Can you work these out from the model? Positions are in its coordinate system, mm. A direction names the side the tool comes from. Round coordinates to 2 decimals unless told otherwise and drop trailing zeros. Loops run counter-clockwise (first coordinate to the right, second up) from the corner with the lowest first, then second, coordinate; pieces in that order, holes last.
(1) Which directions (+Z, -Z, +X, -X, +Y, -Y) give clear straight access to the entire face, cutting with the end or side of a thin tool? Please do faces 1 (the face through (116, 29, 60)), 2 (the face through (62.57, 42.85, 1.18)), 3 (the face through (112, 26, 33.6)).
(2) I want a section at C-C on x = 49. Write out the boundary of the cut face in (y, z), plus the area to 3 significant figures.
(3) Will these pins go through, and if not, where does the flat tip stop? pin 1 Ø4 at (x, z) = (110.5, 112.5) entering from +Y; pin 2 Ø1.5 at (x, z) = (69.5, 46.5) entering from +Y.
(4) If I drill on line 1 along Z through (x, y) = (45.5, 32.5); line 2 along Y through (x, z) = (52, 1.25); line 3 along X through (y, z) = (12, 83), over which ranges is the centre line in solid material (lowest first)?
(5) Thinking about a two-plate mould opening in Z: for faces 4 (the face through (2, 58.4, 32)), 5 (the face through (7.2, 26, 114)), which applies, released by +Z, released by -Z, zero draft, split by the parting line, or undercut?
(6) I want a section at B-B on z = 105.5. Write out the boundary of the cut face in (x, y), plus the area to 3 significant figures.
from build123d import *

# Parameters (mm, degrees)
SKETCH1_W           = 116
SKETCH1_H           = 117.6
BOSS_EXTRUDE1_DEPTH = 2.4
SKETCH2_W           = 116
SKETCH2_H           = 117.6
SKETCH2_W_2         = 111.2
SKETCH2_H_2         = 112.8
BOSS_EXTRUDE2_DEPTH = 56
SKETCH3_R           = 1.5
CUT_EXTRUDE1_DEPTH  = 10
SKETCH7_W           = 4.8
SKETCH7_H           = 4.8
BOSS_EXTRUDE4_DEPTH = 45.6
FILLET2_R           = 2
SKETCH8_R           = 6
CUT_EXTRUDE2_DEPTH  = 10


with BuildPart() as part:
    # Sketch1 → Boss-Extrude1 (new body)
    with BuildSketch(Plane(origin=(0, 0, 0), x_dir=(1, 0, 0), z_dir=(0, 1, 0))):
        with Locations((58, -58.8)):
            Rectangle(SKETCH1_W, SKETCH1_H)
    extrude(amount=BOSS_EXTRUDE1_DEPTH)

    # Sketch2 → Boss-Extrude2 (add)
    with BuildSketch(Plane(origin=(0, 2.4, 0), x_dir=(1, 0, 0), z_dir=(0, 1, 0))):
        with Locations((58, -58.8)):
            Rectangle(SKETCH2_W, SKETCH2_H)
        with Locations((58, -58.8)):
            Rectangle(SKETCH2_W_2, SKETCH2_H_2, mode=Mode.SUBTRACT)
    extrude(amount=BOSS_EXTRUDE2_DEPTH)

    # Sketch3 → Cut-Extrude1 (cut)
    with BuildSketch(Plane(origin=(0, 0, 0), x_dir=(-1, 0, 0), z_dir=(0, 0, -1))):
        with Locations((-64, 42.4)):
            Circle(SKETCH3_R)
        with Locations((-52, 42.4)):
            Circle(SKETCH3_R)
    extrude(amount=-CUT_EXTRUDE1_DEPTH, mode=Mode.SUBTRACT)

    # Sketch7 → Boss-Extrude4 (add)
    with BuildSketch(Plane(origin=(0, 2.4, 0), x_dir=(1, 0, 0), z_dir=(0, 1, 0))):
        with Locations((4.8, -112.8)):
            Rectangle(SKETCH7_W, SKETCH7_H)
        with Locations((4.8, -36)):
            Rectangle(SKETCH7_W, SKETCH7_H)
        with Locations((111.2, -112.8)):
            Rectangle(SKETCH7_W, SKETCH7_H)
        with Locations((111.2, -36)):
            Rectangle(SKETCH7_W, SKETCH7_H)
    extrude(amount=BOSS_EXTRUDE4_DEPTH)

    # Fillet2
    fillet2_edges = [part.edges().sort_by_distance(p)[0] for p in [
        (4.8, 2.4, 38.4),
        (4.8, 2.4, 33.6),
        (111.2, 2.4, 33.6),
        (111.2, 2.4, 38.4),
        (7.2, 25.2, 38.4),
        (7.2, 48, 36),
        (7.2, 25.2, 33.6),
        (7.2, 2.4, 36),
        (108.8, 25.2, 33.6),
        (108.8, 48, 36),
        (108.8, 25.2, 38.4),
        (108.8, 2.4, 36),
        (7.2, 25.2, 110.4),
        (108.8, 25.2, 110.4),
        (4.8, 2.4, 110.4),
        (7.2, 2.4, 112.8),
        (108.8, 2.4, 112.8),
        (111.2, 2.4, 110.4),
    ]]
    fillet(fillet2_edges, radius=FILLET2_R)

    # Sketch8 → Cut-Extrude2 (cut)
    with BuildSketch(Plane(origin=(0, 0, 0), x_dir=(-1, 0, 0), z_dir=(0, 0, -1))):
        with Locations((-58, 60.8)):
            Circle(SKETCH8_R)
    extrude(amount=-CUT_EXTRUDE2_DEPTH, mode=Mode.SUBTRACT)


solid = part.part
Filled sheet:
1. face 1: +Z, -Z, +X, +Y, -Y
1. face 2: -Z
1. face 3: +Y
2. outline: (0, 0) - (58.4, 0) - (58.4, 2.4) - (2.4, 2.4) - (2.4, 115.2) - (58.4, 115.2) - (58.4, 117.6) - (0, 117.6) - close
2. area: 551 mm2
3. pin 1: stops at y = 48
3. pin 2: stops at y = 2.4
4. line 1: z = 0 to 2.4, 115.2 to 117.6
4. line 2: y = 0 to 40.9, 43.9 to 58.4
4. line 3: x = 0 to 2.4, 113.6 to 116
5. face 4: zero draft
5. face 5: undercut
6. outline: (0, 0) - (116, 0) - (116, 58.4) - (113.6, 58.4) - (113.6, 2.4) - (2.4, 2.4) - (2.4, 58.4) - (0, 58.4) - close
6. area: 547 mm2
